```python
from build123d import *

# Parameters (mm, degrees)
F1_DEPTH     = 12.5
F2_R         = 1.9
F2_W         = 2
F2_H         = 5
F3_DEPTH     = 25
F5_T1_DEPTH  = 5
F5_T3_DEPTH  = 5
F5_T5_DEPTH  = 22.8639018857
F5_T7_DEPTH  = 22.8639018857
F5_T12_DEPTH = 25.7278037714
F5_T17_DEPTH = 25.7278037714
F5_T22_DEPTH = 25.7278037714
F5_T27_DEPTH = 25.7278037714
F5_T32_DEPTH = 25.7278037714
F5_T37_DEPTH = 25.7278037714
F5_T42_DEPTH = 25.7278037714
F5_T47_DEPTH = 25.7278037714
F10_SIZE     = 1


# Not quite as in the source:
# - a fillet or chamfer that OpenCascade refuses, or shapes differently, is made with other operations: its cross-section is extruded or revolved along the edge and cut away or added
# - two fillets or chamfers of one size are made in one step


with BuildPart() as f1:
    # F0 (on Top) → F1 (new body, symmetric)
    with BuildSketch(Plane.XY):
        with BuildLine():
            ThreePointArc((-31.711398723, 5), (-30.3486184122, 2.6632855775), (-29.875, 0))
            ThreePointArc((-29.875, 0), (-30.3486184122, -2.6632855775), (-31.711398723, -5))
            Line((-31.711398723, -5), (31.711398723, -5))
            ThreePointArc((31.711398723, -5), (29.875, 0), (31.711398723, 5))
            Line((31.711398723, 5), (4, 5))
            Line((4, 5), (4, 2.4))
            Line((4, 2.4), (-16, 2.4))
            Line((-16, 2.4), (-16, 5))
            Line((-16, 5), (-31.711398723, 5))
        make_face()
    extrude(amount=F1_DEPTH, both=True)

    # F2 (on face) → F3 (cut)
    with BuildSketch(Plane.XZ.offset(5)):
        with Locations((0, 8.5)):
            Circle(F2_R)
        with Locations((0, -8.5)):
            Circle(F2_R)
        with Locations((-17.711398723, 7)):
            Rectangle(F2_W, F2_H)
        with Locations((-17.711398723, -7)):
            Rectangle(F2_W, F2_H)
        with Locations((17.711398723, 7)):
            Rectangle(F2_W, F2_H)
        with Locations((17.711398723, -7)):
            Rectangle(F2_W, F2_H)
        with Locations((-23, 0.5)):
            Circle(F2_R)
        with Locations((23, 0.5)):
            Circle(F2_R)
    extrude(amount=-F3_DEPTH, mode=Mode.SUBTRACT)

    # F5: chamfer of 4 x 1.8652306326 on 10 edges, made by hand

    # F5_s2 → F5_t1 (cut)
    with BuildSketch(Plane.XY.offset(-9.5)):
        Polygon((22.711398723, -5), (18.711398723, -3.1347693674), (18.711398723, -5), align=None)
        Polygon((-22.711398723, -5), (-18.711398723, -3.1347693674), (-18.711398723, -5), align=None)
        Polygon((-18.711398723, 3.1347693674), (-22.711398723, 5), (-18.711398723, 5), align=None)
        Polygon((18.711398723, 3.1347693674), (22.711398723, 5), (18.711398723, 5), align=None)
    extrude(amount=F5_T1_DEPTH, mode=Mode.SUBTRACT)

    # F5_s4 → F5_t3 (cut)
    with BuildSketch(Plane.XY.offset(4.5)):
        Polygon((22.711398723, -5), (18.711398723, -3.1347693674), (18.711398723, -5), align=None)
        Polygon((-22.711398723, -5), (-18.711398723, -3.1347693674), (-18.711398723, -5), align=None)
        Polygon((-18.711398723, 3.1347693674), (-22.711398723, 5), (-18.711398723, 5), align=None)
        Polygon((18.711398723, 3.1347693674), (22.711398723, 5), (18.711398723, 5), align=None)
    extrude(amount=F5_T3_DEPTH, mode=Mode.SUBTRACT)

    # F5_s6 → F5_t5 (cut)
    with BuildSketch(Plane.XY.offset(-22.8639018857)):
        Polygon((8, 5), (4, 3.1347693674), (4, 5), align=None)
    extrude(amount=F5_T5_DEPTH, mode=Mode.SUBTRACT)

    # F5_s8 → F5_t7 (cut)
    with BuildSketch(Plane.XY):
        Polygon((8, 5), (4, 3.1347693674), (4, 5), align=None)
    extrude(amount=F5_T7_DEPTH, mode=Mode.SUBTRACT)


with BuildPart() as f5_tool10:
    # F5_s11 → F5_t12 (new body)
    with BuildSketch(Plane.XY.offset(-19.8639018857)):
        Polygon((22.711398723, -5), (18.711398723, -3.1347693674), (18.711398723, -5), align=None)
    extrude(amount=F5_T12_DEPTH)

    split(bisect_by=Plane.XY.offset(4.5), keep=Keep.TOP)


with BuildPart() as f1_1:
    add(f1.part)

    # F5_t9: cut F5_tool10
    add(f5_tool10.part, mode=Mode.SUBTRACT)


with BuildPart() as f5_tool15:
    # F5_s16 → F5_t17 (new body)
    with BuildSketch(Plane.XY.offset(-5.8639018857)):
        Polygon((22.711398723, -5), (18.711398723, -3.1347693674), (18.711398723, -5), align=None)
    extrude(amount=F5_T17_DEPTH)

    split(bisect_by=Plane.XY.offset(-4.5), keep=Keep.BOTTOM)


with BuildPart() as f1_2:
    add(f1_1.part)

    # F5_t14: cut F5_tool15
    add(f5_tool15.part, mode=Mode.SUBTRACT)


with BuildPart() as f5_tool20:
    # F5_s21 → F5_t22 (new body)
    with BuildSketch(Plane.XY.offset(5.8639018857)):
        Polygon((-22.711398723, -5), (-18.711398723, -3.1347693674), (-18.711398723, -5), align=None)
    extrude(amount=-F5_T22_DEPTH)

    split(bisect_by=Plane.XY.offset(4.5), keep=Keep.TOP)


with BuildPart() as f1_3:
    add(f1_2.part)

    # F5_t19: cut F5_tool20
    add(f5_tool20.part, mode=Mode.SUBTRACT)


with BuildPart() as f5_tool25:
    # F5_s26 → F5_t27 (new body)
    with BuildSketch(Plane.XY.offset(19.8639018857)):
        Polygon((-22.711398723, -5), (-18.711398723, -3.1347693674), (-18.711398723, -5), align=None)
    extrude(amount=-F5_T27_DEPTH)

    split(bisect_by=Plane.XY.offset(-4.5), keep=Keep.BOTTOM)


with BuildPart() as f1_4:
    add(f1_3.part)

    # F5_t24: cut F5_tool25
    add(f5_tool25.part, mode=Mode.SUBTRACT)


with BuildPart() as f5_tool30:
    # F5_s31 → F5_t32 (new body)
    with BuildSketch(Plane.XY.offset(-19.8639018857)):
        Polygon((-18.711398723, 3.1347693674), (-22.711398723, 5), (-18.711398723, 5), align=None)
    extrude(amount=F5_T32_DEPTH)

    split(bisect_by=Plane.XY.offset(4.5), keep=Keep.TOP)


with BuildPart() as f1_5:
    add(f1_4.part)

    # F5_t29: cut F5_tool30
    add(f5_tool30.part, mode=Mode.SUBTRACT)


with BuildPart() as f5_tool35:
    # F5_s36 → F5_t37 (new body)
    with BuildSketch(Plane.XY.offset(5.8639018857)):
        Polygon((18.711398723, 3.1347693674), (22.711398723, 5), (18.711398723, 5), align=None)
    extrude(amount=-F5_T37_DEPTH)

    split(bisect_by=Plane.XY.offset(4.5), keep=Keep.TOP)


with BuildPart() as f1_6:
    add(f1_5.part)

    # F5_t34: cut F5_tool35
    add(f5_tool35.part, mode=Mode.SUBTRACT)


with BuildPart() as f5_tool40:
    # F5_s41 → F5_t42 (new body)
    with BuildSketch(Plane.XY.offset(19.8639018857)):
        Polygon((-18.711398723, 3.1347693674), (-22.711398723, 5), (-18.711398723, 5), align=None)
    extrude(amount=-F5_T42_DEPTH)

    split(bisect_by=Plane.XY.offset(-4.5), keep=Keep.BOTTOM)


with BuildPart() as f1_7:
    add(f1_6.part)

    # F5_t39: cut F5_tool40
    add(f5_tool40.part, mode=Mode.SUBTRACT)


with BuildPart() as f5_tool45:
    # F5_s46 → F5_t47 (new body)
    with BuildSketch(Plane.XY.offset(-5.8639018857)):
        Polygon((18.711398723, 3.1347693674), (22.711398723, 5), (18.711398723, 5), align=None)
    extrude(amount=F5_T47_DEPTH)

    split(bisect_by=Plane.XY.offset(-4.5), keep=Keep.BOTTOM)


with BuildPart() as f1_8:
    add(f1_7.part)

    # F5_t44: cut F5_tool45
    add(f5_tool45.part, mode=Mode.SUBTRACT)

    # F9: F1 across face


with BuildPart() as f1_9:
    add(f1_8.part)
    add(f1_8.part.mirror(Plane(origin=(0.5278701032, -0.3772073921, 12.5), x_dir=(1, 0, 0), z_dir=(0, 0, 1))))

    # F10
    f10_edges = [f1_9.edges().sort_by_distance(p)[0] for p in [
        (29.875, 0, 37.5),
        (29.875, 0, -12.5),
        (-30.348618, 2.663286, 37.5),
        (-30.348618, -2.663286, 37.5),
        (-30.348618, -2.663286, -12.5),
        (-30.348618, 2.663286, -12.5),
    ]]
    chamfer(f10_edges, length=F10_SIZE)


solid = f1_9.part
```
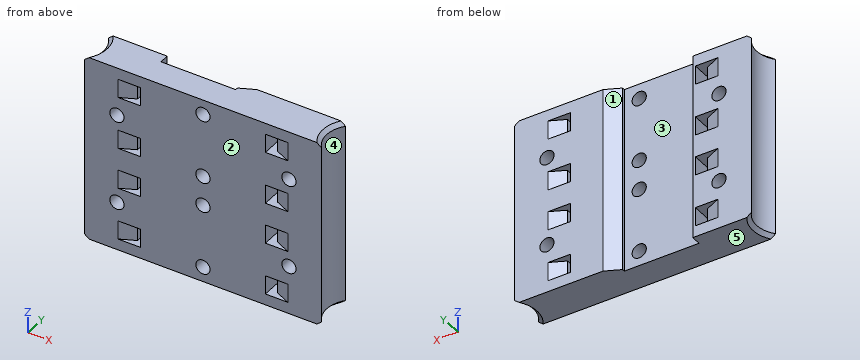
Geometry check sheet. Reference: the model listing, model coordinates, mm. Face numbers are marked on the shaded views. A direction names the side the tool comes from. Coordinates: 2 decimals unless noted, no trailing zeros. Write each loop counter-clockwise with the first axis right and the second up, starting at its lowest first coordinate (ties: lowest second). Pieces come first, ordered by that corner, then holes. Notation, with made-up numbers: M 49.25,75 L 78.25,75 A32 ccw 78.25,108 Z; hole C 34,23.5 d5. An arc over 180 degrees is marked long. Use one line per item in the form item = value. Start each with the question number.
1) Set-up check for the marked faces 1 and 2: record each of +Z, -Z, +X, -X, +Y, -Y from which the full face is reachable in a straight line by a thin tool's end or side.
2) Section check B-B on x = 0. Enter the section's corners in (y, z), and give its area (3 significant figures).
3) Thickness scan on probe 1 along Z at (x, y) = (-23, -0.25); probe 2 along Z at (x, y) = (-17, -2); probe 3 along Z at (x, y) = (0, -2.75). Record the ranges inside material, lowest first. Write a range as from..to.
4) Section check A-A on z = -8.5. Enter the section's corners in (x, y) (3 decimals).
5) Go/stop test with flat-tipped pins: pin 1 Ø1.5 at (y, z) = (1, 19) entering from +X; pin 2 Ø6 at (x, z) = (23, 0.5) entering from -Y; pin 3 Ø4 at (y, z) = (1.5, 32) entering from +X; pin 4 Ø1.5 at (y, z) = (-0.5, 31) entering from -X. Record where each tip stops, or that it passes through.
6) Section check C-C on z = 0.5. Enter the section's corners in (x, y) (3 decimals), and give its area (3 significant figures).
7) Section check D-D on y = -1.75. State how many separate pieces and enclosed holes the cut face has, and give its area (3 significant figures).
8) Release check for a two-part mould opening along Y. For the marked faces 3, 4 and 5 record: pulls with the +Y half, pulls with the -Y half, needs draft (parallel to the pull), parting line crosses it, or undercut.
Responses:
q1.face_1 = +Z, -Z, +Y
q1.face_2 = +Z, -Z, +X, -X, -Y
q2.outline = M -5,-12.5 L 2.4,-12.5 L 2.4,-10.4 L -5,-10.4 Z; M -5,-6.6 L 2.4,-6.6 L 2.4,6.6 L -5,6.6 Z; M -5,10.4 L 2.4,10.4 L 2.4,14.6 L -5,14.6 Z; M -5,18.4 L 2.4,18.4 L 2.4,31.6 L -5,31.6 Z; M -5,35.4 L 2.4,35.4 L 2.4,37.5 L -5,37.5 Z
q2.area = 258 mm2
q3.probe_1 = -12.5..-1.4, 2.4..22.6, 26.4..37.5
q3.probe_2 = -12.5..-9.5, -4.5..4.5, 9.5..15.5, 20.5..29.5, 34.5..37.5
q3.probe_3 = -12.5..-10.4, -6.6..6.6, 10.4..14.6, 18.4..31.6, 35.4..37.5
q4.outline = M -31.711,-5 L -22.711,-5 L -18.711,-3.135 L -18.711,3.135 L -22.711,5 L -31.711,5 A7.725 cw Z; M -16.711,-5 L -1.9,-5 L -1.9,2.4 L -16,2.4 L -16,5 L -16.711,5 Z; M 1.9,-5 L 16.711,-5 L 16.711,5 L 8,5 L 4,3.135 L 4,2.4 L 1.9,2.4 Z; M 18.711,-3.135 L 22.711,-5 L 31.711,-5 A7.725 cw 31.711,5 L 22.711,5 L 18.711,3.135 Z
q5.pin_1 = 30.08
q5.pin_2 = -5
q5.pin_3 = 30.71
q5.pin_4 = -29.98
q6.outline = M -31.711,-5 L -24.9,-5 L -24.9,5 L -31.711,5 A7.725 cw Z; M -21.1,-5 L 21.1,-5 L 21.1,5 L 8,5 L 4,3.135 L 4,2.4 L -16,2.4 L -16,5 L -21.1,5 Z; M 24.9,-5 L 31.711,-5 A7.725 cw 31.711,5 L 24.9,5 Z
q6.area = 477 mm2
q7.separate_pieces = 1
q7.enclosed_holes = 16
q7.area = 2,830 mm2
q8.face_3 = pulls with the +Y half
q8.face_4 = undercut
q8.face_5 = needs draft
